Part model, mm, in its own coordinate system. Face numbers are marked on the shaded views. Coordinates: 2 decimals unless noted, no trailing zeros. Write each loop counter-clockwise with the first axis right and the second up, starting at its lowest first coordinate (ties: lowest second). Pieces come first, ordered by that corner, then holes. Notation, with made-up numbers: M -37,45 L 17,45 A30 ccw 17,74 Z; hole C -30,61 d9. An arc over 180 degrees is marked long. Use a Markdown table: item, result. Add a question column.
Q1. Slice it at C-C on z = -10. Write the cut outline in (x, y).
Q2. Slice it at D-D on x = -37. Write the cut outline in (y, z).
Q3. Slice it at B-B on x = 3. Write the cut outline in (y, z).
Q4. Wall check: L1, parallel to Z at x = 35, y = 6.75; L2, parallel to X at y = 8.75, z = -8.25; L3, parallel to X at y = 1.25, z = -8.25. Give the ranges that are in metal, low to high. Write a range as from..to.
Q5. Mould opens along Z. For the marked faces 1, 2 and 3 say: released by +Z, released by -Z, zero draft, split by the parting line, or undercut.
Q6. Slice it at A-A on y = 8. Write the cut outline in (x, z).
Q7. Pin check, flat tips, straight feed: pin 1 Ø2.5 at (y, z) = (6, 10) entering from +X; pin 2 Ø10 at (x, z) = (-12, -1) entering from +Y; pin 3 Ø4 at (x, z) = (5.5, -9.5) entering from +Y. Stop position of each tip, or through.
from build123d import *

# Parameters (mm, degrees)
F0_W     = 113
F0_H     = 15
F1_DEPTH = 5
F2_W     = 112.967252
F2_H     = 5.205671
F3_DEPTH = 9
F4_R     = 5
F5_W     = 48.795211
F5_H     = 2
F6_DEPTH = 10


with BuildPart() as f1:
    # F0 (on Front) → F1 (new body)
    with BuildSketch(Plane.XZ):
        Rectangle(F0_W, F0_H)
    extrude(amount=-F1_DEPTH)

    # F2 (on face) → F3 (join)
    with BuildSketch(Plane.XZ):
        with Locations((0, 10.102835)):
            Rectangle(F2_W, F2_H)
        with Locations((0, -10.102835)):
            Rectangle(F2_W, F2_H)
    extrude(amount=-F3_DEPTH)

    # F4
    f4_edges = [f1.edges().sort_by_distance(p)[0] for p in [
        (0, 0, 12.705671),
        (0, 0, -12.705671),
    ]]
    fillet(f4_edges, radius=F4_R)

    # F5 (on face) → F6 (cut)
    with BuildSketch(Plane(origin=(0, 0, -12.705671), x_dir=(1, 0, 0), z_dir=(0, 0, -1))):
        with Locations((-0.086021, -8)):
            Rectangle(F5_W, F5_H)
    extrude(amount=-F6_DEPTH, mode=Mode.SUBTRACT)


solid = f1.part
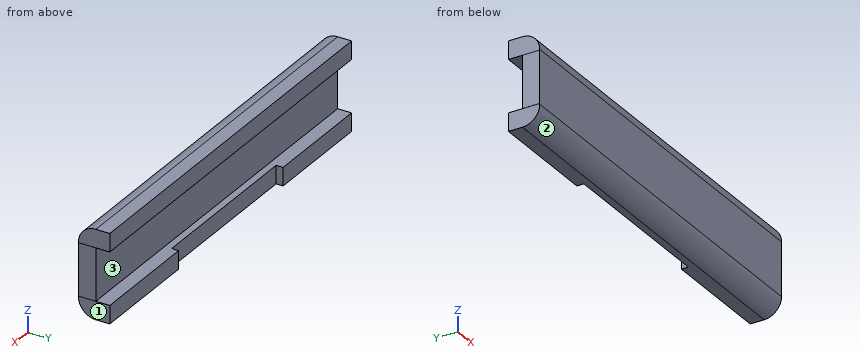
Recorded:
| question | item | result |
|---|---|---|
| 1 | outline | M -56.48,0.56 L 56.48,0.56 L 56.48,9 L 24.31,9 L 24.31,7 L -24.48,7 L -24.48,9 L -56.48,9 Z |
| 2 | outline | M 0,-7.71 A5 ccw 5,-12.71 L 9,-12.71 L 9,-7.5 L 5,-7.5 L 5,7.5 L 9,7.5 L 9,12.71 L 5,12.71 A5 ccw 0,7.71 Z |
| 3 | outline | M 0,-7.71 A5 ccw 5,-12.71 L 7,-12.71 L 7,-7.5 L 5,-7.5 L 5,7.5 L 9,7.5 L 9,12.71 L 5,12.71 A5 ccw 0,7.71 Z |
| 4 | L1 | -12.71..-7.5, 7.5..12.71 |
| 4 | L2 | -56.48..-24.48, 24.31..56.48 |
| 4 | L3 | -56.48..56.48 |
| 5 | face 1 | zero draft |
| 5 | face 2 | released by -Z |
| 5 | face 3 | undercut |
| 6 | outline | M -56.48,-12.71 L -24.48,-12.71 L -24.48,-7.5 L -56.48,-7.5 Z; M -56.48,7.5 L 56.48,7.5 L 56.48,12.71 L -56.48,12.71 Z; M 24.31,-12.71 L 56.48,-12.71 L 56.48,-7.5 L 24.31,-7.5 Z |
| 7 | pin 1 | x = 56.48 |
| 7 | pin 2 | y = 5 |
| 7 | pin 3 | y = 7 |
